```python
from build123d import *

# Parameters (mm, degrees)
ESQUISSE1_R        = 17
BOSS_EXTRU_1_DEPTH = 40
ESQUISSE2_R        = 5
BOSS_EXTRU_2_DEPTH = 3
CONG_1_R           = 1
ESQUISSE3_R        = 18
BOSS_EXTRU_3_DEPTH = 22
CONG_2_R           = 1
BOSS_EXTRU_4_DEPTH = 6
ESQUISSE5_R        = 10
BOSS_EXTRU_5_DEPTH = 11


with BuildPart() as part:
    # Esquisse1 → Boss.-Extru.1 (new body)
    with BuildSketch(Plane.XY):
        Circle(ESQUISSE1_R)
    extrude(amount=BOSS_EXTRU_1_DEPTH)

    # Esquisse2 → Boss.-Extru.2 (add)
    with BuildSketch(Plane.XY.offset(40)):
        Circle(ESQUISSE2_R)
    extrude(amount=BOSS_EXTRU_2_DEPTH)

    # Congé1
    cong_1_edges = [part.edges().sort_by_distance(p)[0] for p in [
        (-17, 0, 40),
    ]]
    fillet(cong_1_edges, radius=CONG_1_R)

    # Esquisse3 → Boss.-Extru.3 (add)
    with BuildSketch(Plane.XY.offset(43)):
        Circle(ESQUISSE3_R)
    extrude(amount=BOSS_EXTRU_3_DEPTH)

    # Congé2
    cong_2_edges = [part.edges().sort_by_distance(p)[0] for p in [
        (-18, 0, 65),
    ]]
    fillet(cong_2_edges, radius=CONG_2_R)

    # Esquisse4 → Boss.-Extru.4 (add)
    with BuildSketch(Plane.XY.offset(65)):
        with BuildLine():
            Line((-13.350159933, -4), (13.350159933, -4))
            ThreePointArc((13.350159933, -4), (17, -1.636663523), (16.336939985, 2.660666256))
            Line((16.336939985, 2.660666256), (5.973560103, 14.294269767))
            ThreePointArc((5.973560103, 14.294269767), (0, 16.972937256), (-5.973560103, 14.294269767))
            Line((-5.973560103, 14.294269767), (-16.336939985, 2.660666256))
            ThreePointArc((-16.336939985, 2.660666256), (-17, -1.636663523), (-13.350159933, -4))
        make_face()
    extrude(amount=BOSS_EXTRU_4_DEPTH)

    # Esquisse5 → Boss.-Extru.5 (add)
    with BuildSketch(Plane.XY.offset(71)):
        with Locations(Location((0, 6, 0), (0, 0, 142.149265436))):
            Circle(ESQUISSE5_R)
    extrude(amount=BOSS_EXTRU_5_DEPTH)


solid = part.part
```
Verification items for the finished model (mm, model axes). A direction names the side the tool comes from. Give positions to 0.01 mm unless a question says otherwise; leave off trailing zeros. Order: outer loops, then holes, each group sorted by start corner. A loop starts at its lowest first (then second) coordinate and runs counter-clockwise, first axis right, second up. Notation, with made-up numbers: M -39.75,23.5 L 18.25,23.5 A16 ccw 18.25,37.5 Z; hole C 9,45 d8. An arc over 180 degrees is marked long. Return JSON: item names as keys, results as strings. Group by question number.
1) Section check B-B on z = 61. Record the cut outline in (x, y), and give its area (3 significant figures).
2) Section check A-A on y = 0. Record the cut outline in (x, z).
3) Go/stop test with flat-tipped pins: pin 1 Ø4 at (x, y) = (-2, -14) entering from -Z; pin 2 Ø8 at (x, z) = (-13.5, 44.5) entering from +Y; pin 3 Ø3 at (y, z) = (10.5, 10) entering from -X; pin 4 Ø4 at (x, y) = (1, -9) entering from +Z. Record where each tip stops, or that it passes through.
4) Section check C-C on z = 6.5. Record the cut outline in (x, y).
5) Scan lines: line 1 (Z direction, x = 16, y = -1.5); line 2 (Y direction, x = -0.5, z = 19.5); line 3 (Z direction, x = -12, y = 9.5). Record each from-to range of solid material in increasing order.
6) Access from +Z, -Z, +X, -X, +Y, -Y to the whole of each face (thin tool, end or side, straight path). Record for faces 1 (the face through (0, 16.2, 71)), 2 (the face through (9.139, 14.334, 19.227)), 3 (the face through (-1.08, -4.88, 41.48)), 4 (the face through (0, -4, 68)).
7) Mould release check, pull along Z, two halves, no side actions. Record for faces 5 (the face through (-4, 4, 40)), 6 (the face through (4, -4, 43)), 7 (the face through (-17.026, -1.578, 67.958)), 8 (the face through (0, -9, 65)): pulls with the +Z half, pulls with the -Z half, needs draft (parallel to the pull), parting line crosses it, or undercut.
Answer block:
{
 "1": {"outline": "C 0,0 d36", "area": "1,020 mm^2"},
 "2": {"outline": "M -18,43 L -5,43 L -5,40 L -16,40 A1 ccw -17,39 L -17,0 L 17,0 L 17,39 A1 ccw 16,40 L 5,40 L 5,43 L 18,43 L 18,64 A1 ccw 17,65 L 17.35,65 L 17.35,71 L 8,71 L 8,82 L -8,82 L -8,71 L -17.35,71 L -17.35,65 L -17,65 A1 ccw -18,64 Z"},
 "3": {"pin 1": "stops at z = 0", "pin 2": "stops at y = 15.29", "pin 3": "stops at x = -14.42", "pin 4": "stops at z = 65"},
 "4": {"outline": "C 0,0 d34"},
 "5": {"line 1": "z = 0 to 40, 43 to 71", "line 2": "y = -16.99 to 16.99", "line 3": "z = 0 to 40, 43 to 65"},
 "6": {"face 1": "+Z, +Y", "face 2": "-Z", "face 3": "none", "face 4": "+Z, +X, -X, -Y"},
 "7": {"face 5": "undercut", "face 6": "undercut", "face 7": "needs draft", "face 8": "pulls with the +Z half"}
}
